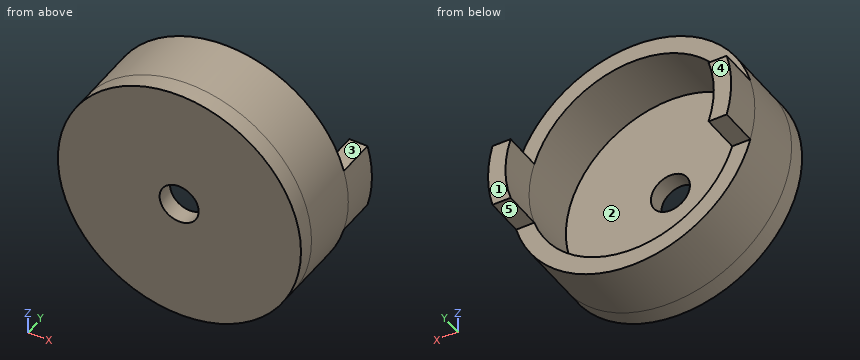
Autodesk Inventor part; units mm, degrees
ref_plane "YZ Plane" through (0, 0, 0) normal (1, 0, 0) x (0, 1, 0)
ref_plane "XZ Plane" through (0, 0, 0) normal (0, 1, 0) x (-1, 0, 0)
ref_plane "XY Plane" through (0, 0, 0) normal (0, 0, 1) x (1, 0, 0)
sketch "Sketch1" plane through (0, 0, 0) normal (0, 1, 0) x (-1, 0, 0)
  circle A0 centre (0, 0) radius 14
  circle A1 centre (0, 0) radius 12
  dimension "d0" = 28
  dimension "d1" = 24
extrude "Extrusion1" add sketch "Sketch1" along normal blind 7
sketch "Sketch2" plane through (0, 7, 0) normal (0, 1, 0) x (1, 0, 0)
  line L0 (14, -3.75) -> (-14, -3.75)
  line L1 (-14, -3.75) -> (-14, 3.75)
  line L2 (-14, 3.75) -> (14, 3.75)
  line L3 (14, 3.75) -> (14, -3.75)
  line L4 (14, -3.75) -> (-14, 3.75) construction
  line L5 (-14, -3.75) -> (14, 3.75) construction
  line L6 (-0.5, 5) -> (0.5, 5)
  line L7 (0.5, 5) -> (0.5, -5)
  line L8 (0.5, -5) -> (-0.5, -5)
  line L9 (-0.5, -5) -> (-0.5, 5)
  line L10 (-0.5, 5) -> (0.5, -5) construction
  line L11 (0.5, 5) -> (-0.5, -5) construction
  circle A0 centre (0, 0) radius 12
  circle A1 centre (0, 0) radius 14
  point P0 (0, 0)
  point P1 (-13.4884, 3.75)
  point P2 (-13.4884, -3.75)
  point P3 (-11.399, -3.75)
  point P4 (-11.399, 3.75)
  point P5 (13.4884, 3.75)
  point P6 (11.399, 3.75)
  point P7 (11.399, -3.75)
  point P8 (13.4884, -3.75)
  dimension "d4" = 28
  dimension "d5" = 7.5
  dimension "d27" = 24
  dimension "d28" = 28
sketch "Sketch3" plane through (0, 0, 0) normal (0, -1, 0) x (1, 0, 0)
  circle A0 centre (0, 0) radius 14
  dimension "d17" = 28
extrude "Extrusion3" add sketch "Sketch3" along normal blind 2
sketch "Sketch5" plane through (0, 0, 0) normal (0, 1, 0) x (1, 0, 0)
  point P0 (0, 0)
  point P1 (-0.0372, -0.1116)
hole "Hole2" at (-0.0372, 0, 0.1116) direction (0, -1, 0) diameter 4.5 end through all
extrude "Extrusion4" add sketch "Sketch2" along normal blind 4.5 contours L0 A0 L2 A1 | A1 L2 A0 L0
properties part number "magneticslotV1"
Verification items for the finished model (mm, model axes). Face numbers are marked on the shaded views. A direction names the side the tool comes from. Round coordinates to 2 decimals unless told otherwise and drop trailing zeros. Loops run counter-clockwise (first coordinate to the right, second up) from the corner with the lowest first, then second, coordinate; pieces in that order, holes last. Notation, with made-up numbers: (49.5, 32) - (87.5, 32) arc R21 cw to (87.5, 36) - close; hole circle Ø3 at (-22, -17). An arc over 180 degrees is marked (long way). Answer in a Markdown table with one row per item. Add a question column.
Q1. Gauge pin test, flat ends, axial feed: pin 1 (2 mm diameter, centred on x = 9.5, y = 9.5, fed in from -Z); pin 2 (2 mm diameter, centred on y = 5, z = 5, fed in from -X); pin 3 (3 mm diameter, centred on x = -2.5, z = -8, fed in from +Y); pin 4 (2 mm diameter, centred on x = 8, y = 4, fed in from -Z). Record the tip position at first contact, or that the pin passes through.
Q2. Section check D-D on z = 7.5. Enter the section's corners in (x, y), plus the area to 3 significant figures.
Q3. Section check C-C on x = -6.25. Enter the section's corners in (y, z), plus the area to 3 significant figures.
Q4. Section check A-A on y = 10.25. Enter the section's corners in (x, z), plus the area to 3 significant figures.
Q5. Release check for a two-part mould opening along X. For the marked faces 1 and 2 record: pulls with the +X half, pulls with the -X half, needs draft (parallel to the pull), parting line crosses it, or undercut.
Q6. Section check B-B on z = 0. Enter the section's corners in (x, y).
Q7. Material ranges on line 1 (Z direction, x = 0, y = 2.25); line 2 (Y direction, x = 7.75, z = 7), recorded low to high.
Q8. Tool access check on the marked faces 3, 4 and 5. Record the directions out of +Z, -Z, +X, -X, +Y, -Y that give a thin tool (end or side, any length) a straight path to the whole face; none if there is none.
Found:
| question | item | result |
|---|---|---|
| 1 | pin 1 | passes through |
| 1 | pin 2 | stops at x = -13.42 |
| 1 | pin 3 | stops at y = 0 |
| 1 | pin 4 | stops at z = -12.12 |
| 2 | outline | (-11.82, -2) - (11.82, -2) - (11.82, 7) - (9.37, 7) - (9.37, 0) - (-9.37, 0) - (-9.37, 7) - (-11.82, 7) - close |
| 2 | area | 81.6 mm² |
| 3 | outline | (-2, -12.53) - (7, -12.53) - (7, -10.24) - (0, -10.24) - (0, 10.24) - (7, 10.24) - (7, 12.53) - (-2, 12.53) - close |
| 3 | area | 82.1 mm² |
| 4 | outline | (-13.49, -3.75) - (-11.4, -3.75) arc R12 cw to (-11.4, 3.75) - (-13.49, 3.75) arc R14 ccw to start; (11.4, -3.75) - (13.49, -3.75) arc R14 ccw to (13.49, 3.75) - (11.4, 3.75) arc R12 cw to start |
| 4 | area | 30.4 mm² |
| 5 | face 1 | needs draft |
| 5 | face 2 | undercut |
| 6 | outline | (-14, -2) - (-2.28, -2) - (-2.28, 0) - (-12, 0) - (-12, 11.5) - (-14, 11.5) - close; (2.21, -2) - (14, -2) - (14, 11.5) - (12, 11.5) - (12, 0) - (2.21, 0) - close |
| 7 | line 1 | z = -14 to -12, 12 to 14 |
| 7 | line 2 | y = -2 to 0 |
| 8 | face 3 | +Z, +X, -X, +Y |
| 8 | face 4 | +Z, -Z, +X, -X, +Y |
| 8 | face 5 | -Z, +X, -X, +Y |
